For this review, take the finished solid that the model builds, in its own axes (mm). Coordinates: 2 decimals unless noted, no trailing zeros. Write each loop counter-clockwise with the first axis right and the second up, starting at its lowest first coordinate (ties: lowest second). Pieces come first, ordered by that corner, then holes. Notation, with made-up numbers: (54, 33.25) - (88, 33.25) arc R19 cw to (88, 38.25) - close; hole circle Ø11 at (-0.75, 59). An arc over 180 degrees is marked (long way). Write each question's results on one line, items separated by ' | '.
from build123d import *

# Parameters (mm, degrees)
SKETCH_1_W                       = 580
SKETCH_1_H                       = 540
EXTRUDE_1_DEPTH                  = 100
SHELL_1_T                        = -20
SKETCH_2_W                       = 235
SKETCH_2_H                       = 200
CUT_EXTRUDE_1_DEPTH              = 43
PATTERN_LINEAR_1_COUNT           = 2
PATTERN_LINEAR_1_PITCH           = 305
PATTERN_LINEAR_2_COUNT           = 2
PATTERN_LINEAR_2_PITCH           = 300
PATTERN_LINEAR_3_COPY_1_SKETCH_W = 235
PATTERN_LINEAR_3_COPY_1_SKETCH_H = 200
PATTERN_LINEAR_3_COPY_1_DEPTH    = 43
PATTERN_LINEAR_3_COPY_2_SKETCH_W = 235
PATTERN_LINEAR_3_COPY_2_SKETCH_H = 200
PATTERN_LINEAR_3_COPY_2_DEPTH    = 43
SKETCH_4_W                       = 260
SKETCH_4_H                       = 80
CUT_EXTRUDE_2_DEPTH              = 549
SKETCH_6_W                       = 80
SKETCH_6_H                       = 220
CUT_EXTRUDE_3_DEPTH              = 614
SKETCH_8_W                       = 120
SKETCH_8_H                       = 60
CUT_EXTRUDE_4_DEPTH              = 614
SKETCH_10_W                      = 120
SKETCH_10_H                      = 60
CUT_EXTRUDE_5_DEPTH              = 614
SKETCH_12_W                      = 60
SKETCH_12_H                      = 120
CUT_EXTRUDE_6_DEPTH              = 602
SKETCH_13_W                      = 60
SKETCH_13_H                      = 120
CUT_EXTRUDE_7_DEPTH              = 602
SKETCH_15_W                      = 30
SKETCH_15_H                      = 500
CUT_EXTRUDE_8_DEPTH              = 66
SKETCH_18_W                      = 235
SKETCH_18_H                      = 60
CUT_EXTRUDE_11_DEPTH             = 41
SKETCH_21_W                      = 235
SKETCH_21_H                      = 60
CUT_EXTRUDE_13_DEPTH             = 72


with BuildPart() as part:
    # 草图1 → 凸台-拉伸1 (new body)
    with BuildSketch(Plane.XY):
        with Locations((290, 270)):
            Rectangle(SKETCH_1_W, SKETCH_1_H)
    extrude(amount=EXTRUDE_1_DEPTH)

    # 抽壳1
    shell_1_openings = [part.faces().sort_by_distance(p)[0] for p in [
        (290, 270, 100),
    ]]
    offset(amount=SHELL_1_T, openings=shell_1_openings, kind=Kind.INTERSECTION)

    # 草图2 → 切除-拉伸1 (cut)
    with BuildSketch(Plane.XY.offset(20)):
        with Locations((442.5, 120)):
            Rectangle(SKETCH_2_W, SKETCH_2_H)
    cut_extrude_1 = extrude(amount=-CUT_EXTRUDE_1_DEPTH, mode=Mode.SUBTRACT)

    # 阵列(线性)1: 切除-拉伸1 ×2
    with Locations(*[(-i * PATTERN_LINEAR_1_PITCH, 0, 0) for i in range(1, PATTERN_LINEAR_1_COUNT)]):
        add(cut_extrude_1, mode=Mode.SUBTRACT)

    # 阵列(线性)2: 切除-拉伸1 ×2
    with Locations(*[(0, i * PATTERN_LINEAR_2_PITCH, 0) for i in range(1, PATTERN_LINEAR_2_COUNT)]):
        add(cut_extrude_1, mode=Mode.SUBTRACT)

    # 阵列(线性)3 copy 1 sketch → 阵列(线性)3 copy 1 (cut)
    with BuildSketch(Plane(origin=(-305, 300, 20), x_dir=(1, 0, 0), z_dir=(0, 0, 1))):
        with Locations((442.5, 120)):
            Rectangle(PATTERN_LINEAR_3_COPY_1_SKETCH_W, PATTERN_LINEAR_3_COPY_1_SKETCH_H)
    extrude(amount=-PATTERN_LINEAR_3_COPY_1_DEPTH, mode=Mode.SUBTRACT)

    # 阵列(线性)3 copy 2 sketch → 阵列(线性)3 copy 2 (cut)
    with BuildSketch(Plane(origin=(0, 300, 20), x_dir=(1, 0, 0), z_dir=(0, 0, 1))):
        with Locations((442.5, 120)):
            Rectangle(PATTERN_LINEAR_3_COPY_2_SKETCH_W, PATTERN_LINEAR_3_COPY_2_SKETCH_H)
    extrude(amount=-PATTERN_LINEAR_3_COPY_2_DEPTH, mode=Mode.SUBTRACT)

    # 草图4 → 切除-拉伸2 (cut)
    with BuildSketch(Plane.XZ):
        with Locations((290, 60)):
            Rectangle(SKETCH_4_W, SKETCH_4_H)
    extrude(amount=-CUT_EXTRUDE_2_DEPTH, mode=Mode.SUBTRACT)

    # 草图6 → 切除-拉伸3 (cut)
    with BuildSketch(Plane(origin=(580, 0, 0), x_dir=(0, 0, -1), z_dir=(1, 0, 0))):
        with Locations((-60, 270)):
            Rectangle(SKETCH_6_W, SKETCH_6_H)
    extrude(amount=-CUT_EXTRUDE_3_DEPTH, mode=Mode.SUBTRACT)

    # 草图8 → 切除-拉伸4 (cut)
    with BuildSketch(Plane.XZ):
        with Locations((80, 50)):
            Rectangle(SKETCH_8_W, SKETCH_8_H)
    extrude(amount=-CUT_EXTRUDE_4_DEPTH, mode=Mode.SUBTRACT)

    # 草图10 → 切除-拉伸5 (cut)
    with BuildSketch(Plane.XZ):
        with Locations((500, 50)):
            Rectangle(SKETCH_10_W, SKETCH_10_H)
    extrude(amount=-CUT_EXTRUDE_5_DEPTH, mode=Mode.SUBTRACT)

    # 草图12 → 切除-拉伸6 (cut)
    with BuildSketch(Plane(origin=(580, 0, 0), x_dir=(0, 0, -1), z_dir=(1, 0, 0))):
        with Locations((-50, 460)):
            Rectangle(SKETCH_12_W, SKETCH_12_H)
    extrude(amount=-CUT_EXTRUDE_6_DEPTH, mode=Mode.SUBTRACT)

    # 草图13 → 切除-拉伸7 (cut)
    with BuildSketch(Plane(origin=(580, 0, 0), x_dir=(0, 0, -1), z_dir=(1, 0, 0))):
        with Locations((-50, 80)):
            Rectangle(SKETCH_13_W, SKETCH_13_H)
    extrude(amount=-CUT_EXTRUDE_7_DEPTH, mode=Mode.SUBTRACT)

    # 草图15 → 切除-拉伸8 (cut)
    with BuildSketch(Plane.XY.offset(20)):
        with Locations((290, 270)):
            Rectangle(SKETCH_15_W, SKETCH_15_H)
    extrude(amount=-CUT_EXTRUDE_8_DEPTH, mode=Mode.SUBTRACT)

    # 草图18 → 切除-拉伸11 (cut)
    with BuildSketch(Plane.XY.offset(20)):
        with Locations((137.5, 270)):
            Rectangle(SKETCH_18_W, SKETCH_18_H)
    extrude(amount=-CUT_EXTRUDE_11_DEPTH, mode=Mode.SUBTRACT)

    # 草图21 → 切除-拉伸13 (cut)
    with BuildSketch(Plane.XY.offset(20)):
        with Locations((442.5, 270)):
            Rectangle(SKETCH_21_W, SKETCH_21_H)
    extrude(amount=-CUT_EXTRUDE_13_DEPTH, mode=Mode.SUBTRACT)


solid = part.part
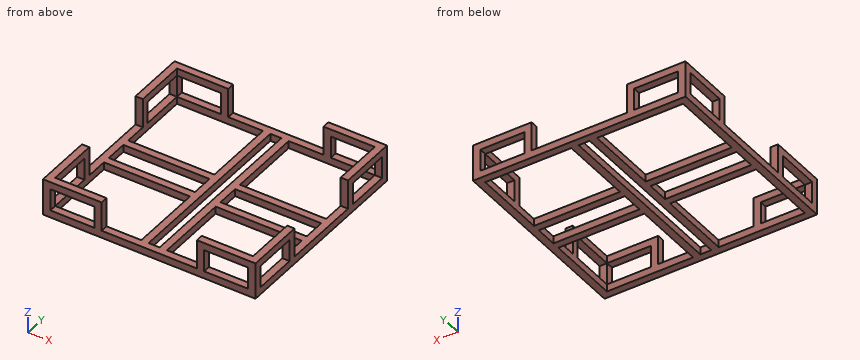
Q1. Take a section at A-A on x = 245. State the section outline as (y, z) points.
Results found:
outline: (0, 0) - (20, 0) - (20, 20) - (0, 20) - close; (220, 0) - (240, 0) - (240, 20) - (220, 20) - close; (300, 0) - (320, 0) - (320, 20) - (300, 20) - close; (520, 0) - (540, 0) - (540, 20) - (520, 20) - close
Q2. Wall thickness on line 1 along Y through (x, z) = (217, 17.5); line 2 along Y through (x, z) = (429, 55); line 3 along X through (y, z) = (147, 93): over which ranges is each line inside the solid? List them lowest first. Write a range as from..to.
Results found:
line 1: 0..20, 220..240, 300..320, 520..540 | line 2: 0..20, 520..540 | line 3: 0..20, 560..580
Q3. For pin 1 (5 mm diameter, centred on x = 415.5, y = 319.5, fed in from +Z); pin 2 (8 mm diameter, centred on x = 398, z = 24.5, fed in from -Y); pin 3 (10 mm diameter, centred on y = 11.5, z = 35, fed in from -X), all flat-tipped, find the tip position at first contact; note any pin that passes through.
Results found:
pin 1: z = 20 | pin 2: through | pin 3: x = 0
Q4. Take a section at C-C on x = 117.5. State the section outline as (y, z) points.
Results found:
outline: (0, 0) - (20, 0) - (20, 20) - (0, 20) - close; (0, 80) - (20, 80) - (20, 100) - (0, 100) - close; (220, 0) - (240, 0) - (240, 20) - (220, 20) - close; (300, 0) - (320, 0) - (320, 20) - (300, 20) - close; (520, 0) - (540, 0) - (540, 20) - (520, 20) - close; (520, 80) - (540, 80) - (540, 100) - (520, 100) - close
Q5. Take a section at B-B on y = 345.5. State the section outline as (x, z) points.
Results found:
outline: (0, 0) - (20, 0) - (20, 20) - (0, 20) - close; (255, 0) - (275, 0) - (275, 20) - (255, 20) - close; (305, 0) - (325, 0) - (325, 20) - (305, 20) - close; (560, 0) - (580, 0) - (580, 20) - (560, 20) - close
Q6. Take a section at D-D on y = 469. State the section outline as (x, z) points, plus the area to 3 significant figures.
Results found:
outline: (0, 0) - (20, 0) - (20, 20) - (0, 20) - close; (0, 80) - (20, 80) - (20, 100) - (0, 100) - close; (255, 0) - (275, 0) - (275, 20) - (255, 20) - close; (305, 0) - (325, 0) - (325, 20) - (305, 20) - close; (560, 0) - (580, 0) - (580, 20) - (560, 20) - close; (560, 80) - (580, 80) - (580, 100) - (560, 100) - close | area: 2,400 mm2
